```python
from build123d import *

# Parameters (mm, degrees)
F1_DEPTH = 25
F3_DEPTH = 25


with BuildPart() as f1:
    # F0 (on Top) → F1 (new body)
    with BuildSketch(Plane.XY):
        with BuildLine():
            Line((325, 560), (-325, 560))
            ThreePointArc((-325, 560), (-360.355339, 545.355339), (-375, 510))
            Line((-375, 510), (-375, -510))
            ThreePointArc((-375, -510), (-360.355339, -545.355339), (-325, -560))
            Line((-325, -560), (325, -560))
            ThreePointArc((325, -560), (360.355339, -545.355339), (375, -510))
            Line((375, -510), (375, 510))
            ThreePointArc((375, 510), (360.355339, 545.355339), (325, 560))
        make_face()
    extrude(amount=F1_DEPTH)

    # F2 (on face) → F3 (cut)
    with BuildSketch(Plane.XY.offset(25)):
        with BuildLine():
            Line((215, 450), (-215, 450))
            ThreePointArc((-215, 450), (-250.355339, 435.355339), (-265, 400))
            Line((-265, 400), (-265, -400))
            ThreePointArc((-265, -400), (-250.355339, -435.355339), (-215, -450))
            Line((-215, -450), (215, -450))
            ThreePointArc((215, -450), (250.355339, -435.355339), (265, -400))
            Line((265, -400), (265, 400))
            ThreePointArc((265, 400), (250.355339, 435.355339), (215, 450))
        make_face()
    extrude(amount=-F3_DEPTH, mode=Mode.SUBTRACT)


solid = f1.part
```
Design review of the part built by this model. Coordinates are the model's own, in mm. A direction names the side the tool comes from. Coordinates: 2 decimals unless noted, no trailing zeros. Order: outer loops, then holes, each group sorted by start corner. A loop starts at its lowest first (then second) coordinate and runs counter-clockwise, first axis right, second up. Notation, with made-up numbers: (85.25, -25.75) - (118.25, -25.75) arc R29 ccw to (118.25, 2.25) - close; hole circle Ø7 at (41, 33). An arc over 180 degrees is marked (long way). Answer in a Markdown table with one row per item.
(1) The part is to be moulded in two halves that separate along X. For faces 1 (the cylindrical face through (-360.742, -544.964, 12.325)), 2 (the cylindrical face through (-250.742, -434.964, 12.675)), 3 (the cylindrical face through (360.742, 544.964, 12.325)), say which applies: released by +X, released by -X, zero draft, split by the parting line, or undercut.
Checked values:
| item | result |
|---|---|
| face 1 | released by -X |
| face 2 | undercut |
| face 3 | released by +X |
(2) Wall thickness on line 1 along X through (y, z) = (137.5, 4); line 2 along Y through (x, z) = (146, 23.25); line 3 along X through (y, z) = (-439.5, 6): over which ranges is each line inside the solid? List them lowest first. Write a range as from..to.
Checked values:
| item | result |
|---|---|
| line 1 | -375..-265, 265..375 |
| line 2 | -560..-450, 450..560 |
| line 3 | -375..-245.66, 245.66..375 |
(3) Consider section A-A on x = -54. State the section outline as (y, z) points, plus the area to 3 significant figures.
Checked values:
| item | result |
|---|---|
| outline | (-560, 0) - (-450, 0) - (-450, 25) - (-560, 25) - close; (450, 0) - (560, 0) - (560, 25) - (450, 25) - close |
| area | 5,500 mm^2 |
(4) Consider section C-C on z = 12.5. State the section outline as (x, y) points, plus the area to 3 significant figures.
Checked values:
| item | result |
|---|---|
| outline | (-375, -510) arc R50 ccw to (-325, -560) - (325, -560) arc R50 ccw to (375, -510) - (375, 510) arc R50 ccw to (325, 560) - (-325, 560) arc R50 ccw to (-375, 510) - close; hole (-265, -400) arc R50 ccw to (-215, -450) - (215, -450) arc R50 ccw to (265, -400) - (265, 400) arc R50 ccw to (215, 450) - (-215, 450) arc R50 ccw to (-265, 400) - close |
| area | 363,000 mm^2 |
(5) Consider section B-B on y = -143.5. State the section outline as (x, z) points, plus the area to 3 significant figures.
Checked values:
| item | result |
|---|---|
| outline | (-375, 0) - (-265, 0) - (-265, 25) - (-375, 25) - close; (265, 0) - (375, 0) - (375, 25) - (265, 25) - close |
| area | 5,500 mm^2 |
(6) For faces 4 (the flat face through (-339, 8, 0)), 5 (the cylindrical face through (250.742, 434.964, 12.675)), list the 3-axis set-ups (+Z, -Z, +X, -X, +Y, -Y) from which the entire face can be reached by the end or side of a thin tool; tool diameter is ignored.
Checked values:
| item | result |
|---|---|
| face 4 | -Z, +X, -X, +Y, -Y |
| face 5 | +Z, -Z |
